Read the model definition and answer for the solid it produces. Units are mm, in the model's axes. Coordinates: 2 decimals unless noted, no trailing zeros. Use CSV: the item, a comma, the result in double quotes.
from build123d import *

# Parameters (mm, degrees)
SKETCH1_W      = 20
SKETCH1_H      = 20
EXTRUDE1_DEPTH = 300
SKETCH2_R      = 2.266666667
SKETCH2_W      = 1.866666667
SKETCH2_H      = 1.866666667
EXTRUDE2_DEPTH = 301.333148354
FILLET1_R      = 1.333333333


with BuildPart() as part:
    # Sketch1 → Extrude1 (new body)
    with BuildSketch(Plane(origin=(0, 0, 0), x_dir=(1, 0, 0), z_dir=(0, 1, 0))):
        Rectangle(SKETCH1_W, SKETCH1_H)
    extrude(amount=EXTRUDE1_DEPTH)

    # Sketch2 → Extrude2 (cut, through all)
    with BuildSketch(Plane(origin=(0, 300, 0), x_dir=(1, 0, 0), z_dir=(0, 1, 0))):
        with Locations(Location((0, 0, 0), (0, 0, 270))):
            Circle(SKETCH2_R)
        Polygon((8.666666667, 3), (11.333333333, 3), (11.333333333, -3), (8.666666667, -3), (8.666666667, -5.466666667), (6.409475708, -5.466666667), (4.133333333, -3.190524292), (4.133333333, 3.190524292), (6.409475708, 5.466666667), (8.666666667, 5.466666667), align=None)
        with Locations((7.733333334, 7.733333334)):
            Rectangle(SKETCH2_W, SKETCH2_H)
        Polygon((-3.190524292, 4.133333333), (-5.466666667, 6.409475708), (-5.466666667, 8.666666667), (-3, 8.666666667), (-3, 11.333333333), (3, 11.333333333), (3, 8.666666667), (5.466666667, 8.666666667), (5.466666667, 6.409475708), (3.190524292, 4.133333333), align=None)
        with Locations((7.733333334, -7.733333334)):
            Rectangle(SKETCH2_W, SKETCH2_H)
        with Locations((-7.733333334, 7.733333334)):
            Rectangle(SKETCH2_W, SKETCH2_H)
        with Locations((-7.733333334, -7.733333334)):
            Rectangle(SKETCH2_W, SKETCH2_H)
        Polygon((-6.409475708, -5.466666667), (-8.666666667, -5.466666667), (-8.666666667, -3), (-11.333333333, -3), (-11.333333333, 3), (-8.666666667, 3), (-8.666666667, 5.466666667), (-6.409475708, 5.466666667), (-4.133333333, 3.190524292), (-4.133333333, -3.190524292), align=None)
        Polygon((3.190524292, -4.133333333), (-3.190524292, -4.133333333), (-5.466666667, -6.409475708), (-5.466666667, -8.666666667), (-3, -8.666666667), (-3, -11.333333333), (3, -11.333333333), (3, -8.666666667), (5.466666667, -8.666666667), (5.466666667, -6.409475708), align=None)
    extrude(amount=-EXTRUDE2_DEPTH, mode=Mode.SUBTRACT)

    # Fillet1
    fillet1_edges = [part.edges().sort_by_distance(p)[0] for p in [
        (10, 150, 10),
        (-10, 150, 10),
        (-10, 150, -10),
        (10, 150, -10),
    ]]
    fillet(fillet1_edges, radius=FILLET1_R)


solid = part.part
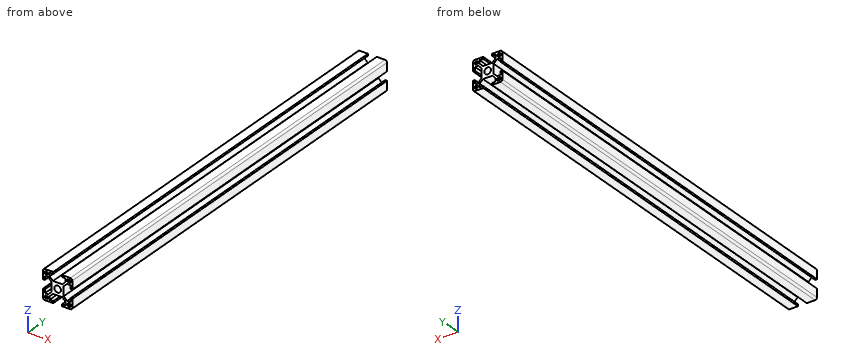
1. Each of these flat-tipped pins is pushed along its axis until it touches: pin 1 Ø1.5 at (x, y) = (-9.5, 179.5) entering from -Z; pin 2 Ø0.7 at (y, z) = (185.5, 9.5) entering from +X; pin 3 Ø1 at (y, z) = (179.5, -1.5) entering from +X. Where does it stop, or does it pass through?
Solutions:
pin 1,"stops at z = -10"
pin 2,"stops at x = 9.91"
pin 3,"stops at x = 4.13"
2. Find the intervals of material crossed by line 1 along X through (y, z) = (126, 7.75); line 2 along X through (y, z) = (235, 0), in increasing order.
Solutions:
line 1,"x = -10 to -8.67, -6.8 to -5.47, 5.47 to 6.8, 8.67 to 10"
line 2,"x = -4.13 to -2.27, 2.27 to 4.13"
3. A cutting plane is placed at A-A (y = 83). Give the number of separate pieces and of enclosed holes in the cut face, and give its area (3 significant figures).
Solutions:
separate pieces,"1"
enclosed holes,"5"
area,"159 mm^2"
